Print and shaded views of the part. All mm, measured from the part's lowest x, y and z. A direction names the side the tool comes from. Round coordinates to 2 decimals unless told otherwise and drop trailing zeros. Loops run counter-clockwise (first coordinate to the right, second up) from the corner with the lowest first, then second, coordinate; pieces in that order, holes last. Notation, with made-up numbers: (6.5, 52.5) -> (23.5, 52.5) arc R19 ccw to (23.5, 82.5) -> close; hole circle Ø1 at (-32, 5.25). An arc over 180 degrees is marked (long way). Answer as CSV lines item,"result".
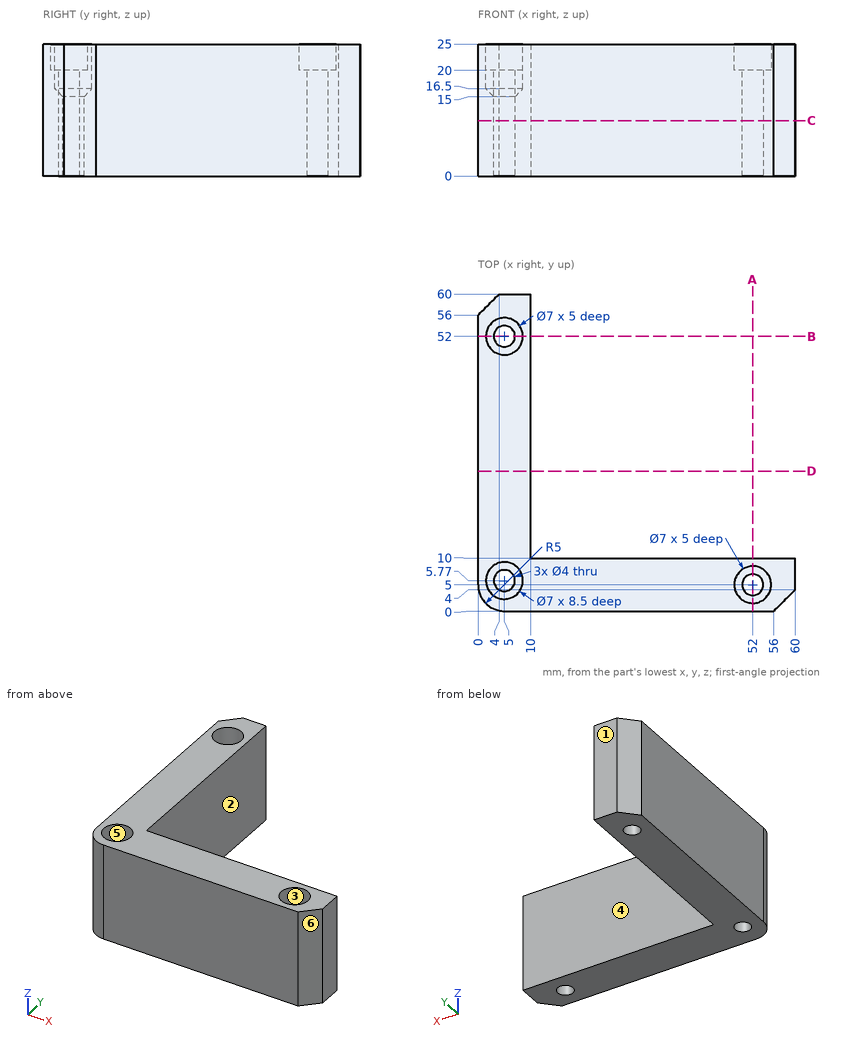
Q1. Saw through at D-D, the plane y = 26.5. Write the cut outline in (x, z), then the cut area to 3 significant figures.
Geometry results:
outline,"(0, 0) -> (10, 0) -> (10, 25) -> (0, 25) -> close"
area,"250 mm2"
Q2. Drop flat-ended pins along their axis: P1, Ø3, axis at x = 5, y = 52, coming from the +Z side; P2, Ø5.5, axis at x = 5, y = 5.77, coming from the +Z side; P3, Ø4, axis at x = 23, z = 11.5, coming from the +Y side; P4, Ø12.5, axis at y = 32.5, z = 17.5, coming from the +X side. Give the stop position or say it passes through.
Geometry results:
P1,"through"
P2,"z = 15.75"
P3,"y = 10"
P4,"x = 10"
Q3. Saw through at A-A, the plane x = 52. Write the cut outline in (y, z).
Geometry results:
outline,"(0, 0) -> (3, 0) -> (3, 20) -> (1.5, 20) -> (1.5, 25) -> (0, 25) -> close; (7, 0) -> (10, 0) -> (10, 25) -> (8.5, 25) -> (8.5, 20) -> (7, 20) -> close"
Q4. Two-plate mould, pull along Y, no slides. Class the marked faces 1, 2 and 3: pulls with the +Y half, pulls with the -Y half, needs draft (parallel to the pull), parting line crosses it, or undercut.
Geometry results:
face 1,"pulls with the +Y half"
face 2,"needs draft"
face 3,"undercut"
Q5. Which spindle directions (+Z, -Z, +X, -X, +Y, -Y) get a long thin tool onto all of the face, cutting with end or side? Do the marked faces 4, 5 and 6. Say none if no direction does.
Geometry results:
face 4,"+Z, -Z, +X, +Y"
face 5,"+Z"
face 6,"+Z, -Z, +X, -Y"
Q6. Drill centre line: line 1 along Y through (x, z) = (12.5, 9.25). Where is it in solid material? Low to high.
Geometry results:
line 1,"0 to 10"
Q7. Saw through at C-C, the plane z = 10.5. Write the cut outline in (x, y).
Geometry results:
outline,"(0, 5) arc R5 ccw to (5, 0) -> (56, 0) -> (60, 4) -> (60, 10) -> (10, 10) -> (10, 60) -> (4, 60) -> (0, 56) -> close; hole circle Ø4 at (5, 5.77); hole circle Ø4 at (5, 52); hole circle Ø4 at (52, 5)"
